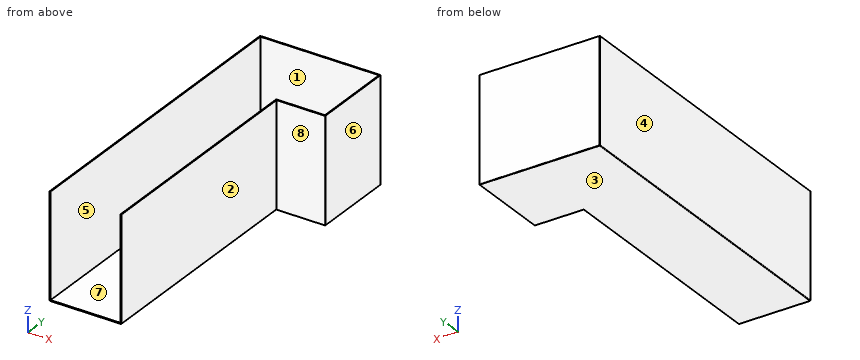
from build123d import *

# Parameters (mm, degrees)
F1_DEPTH = 426
F3_DEPTH = 4
F4_R     = 2


# Not quite as in the source:
# - a feature names something its author has since deleted; it is built from what else it names


with BuildPart() as f1:
    # F0 (on Top) → F1 (new body)
    with BuildSketch(Plane.XY):
        Polygon((-200, -343), (0, -343), (0, 0), (-495, 0), (-495, -1303), (-491, -1303), (-491, -4), (-4, -4), (-4, -339), (-204, -339), (-204, -1303), (-200, -1303), align=None)
    extrude(amount=F1_DEPTH)

    # F2 (on Top) → F3 (join)
    with BuildSketch(Plane.XY):
        Polygon((0, 0), (-495, 0), (-495, -1303), (-200, -1303), (-200, -343), (0, -343), align=None)
    extrude(amount=-F3_DEPTH)

    # F4
    f4_edges = [f1.edges().sort_by_distance(p)[0] for p in [
        (-200, -823, -4),
        (-495, -651.5, -4),
        (-247.5, 0, -4),
        (-495, 0, 211),
        (0, -343, 211),
        (0, 0, 211),
    ]]
    fillet(f4_edges, radius=F4_R)


solid = f1.part
Part model, mm, in its own coordinate system. Face numbers are marked on the shaded views. A direction names the side the tool comes from. Coordinates: 2 decimals unless noted, no trailing zeros. Order: outer loops, then holes, each group sorted by start corner. A loop starts at its lowest first (then second) coordinate and runs counter-clockwise, first axis right, second up. Notation, with made-up numbers: (0.25, 47.25) - (49.25, 47.25) arc R26 cw to (49.25, 78.25) - close; hole circle Ø7 at (-6.5, 18). An arc over 180 degrees is marked (long way). Use CSV: the item, a comma, the result in double quotes.
Item 1: Saw through at B-B on y = -1186.5. Give the cut face in (x, z), and give its area (3 significant figures).
Solved:
outline,"(-495, -2) arc R2 ccw to (-493, -4) - (-202, -4) arc R2 ccw to (-200, -2) - (-200, 426) - (-204, 426) - (-204, 0) - (-491, 0) - (-491, 426) - (-495, 426) - close"
area,"4,590 mm²"
Item 2: 3-axis set-ups, long thin cutter, end or side, ignore diameter. For the marked faces 1, 2, 3, 4 and 5: which of +Z, -Z, +X, -X, +Y, -Y reach the whole face in a straight line?
Solved:
face 1,"+Z"
face 2,"+Z, -Z, +X, -Y"
face 3,"-Z, +X, -X, +Y, -Y"
face 4,"+Z, -Z, -X, +Y, -Y"
face 5,"+Z, -Y"
Item 3: Saw through at C-C on z = 46. Give the cut face in (x, y).
Solved:
outline,"(-495, -1303) - (-491, -1303) - (-491, -4) - (-4, -4) - (-4, -339) - (-204, -339) - (-204, -1303) - (-200, -1303) - (-200, -343) - (-2, -343) arc R2 ccw to (0, -341) - (0, -2) arc R2 ccw to (-2, 0) - (-493, 0) arc R2 ccw to (-495, -2) - close"
Item 4: Saw through at D-D on y = -302.5. Give the cut face in (x, z), and give its area (3 significant figures).
Solved:
outline,"(-495, -2) arc R2 ccw to (-493, -4) - (0, -4) - (0, 426) - (-4, 426) - (-4, 0) - (-491, 0) - (-491, 426) - (-495, 426) - close"
area,"5,390 mm²"
Item 5: Saw through at A-A on x = -33. Give the cut face in (y, z).
Solved:
outline,"(-343, -4) - (-2, -4) arc R2 ccw to (0, -2) - (0, 426) - (-4, 426) - (-4, 0) - (-339, 0) - (-339, 426) - (-343, 426) - close"
Item 6: Drop flat-ended pins along their axis: P1, Ø2, axis at x = -375.5, y = -560, coming from the +Z side; P2, Ø4, axis at x = -236.5, z = 368.5, coming from the -Y side; P3, Ø1.5, axis at y = -1145, z = 214.5, coming from the +X side. Give the stop position or say it passes through.
Solved:
P1,"stops at z = 0"
P2,"stops at y = -4"
P3,"stops at x = -200"
Item 7: Mould opens along Y. For the marked faces 6, 7 and 8 say: +Y half, -Y half, draft (parallel to the pull), parting line (faces both ways), or undercut.
Solved:
face 6,"draft"
face 7,"undercut"
face 8,"-Y half"
Item 8: Probe probe 1 along X at (y, z) = (-614.5, 182); probe 2 along Y at (x, z) = (-156.5, 254); probe 3 along Y at (x, z) = (-361, 308). List the from-to ranges inside material, lowest first.
Solved:
probe 1,"x = -495 to -491, -204 to -200"
probe 2,"y = -343 to -339, -4 to 0"
probe 3,"y = -4 to 0"
